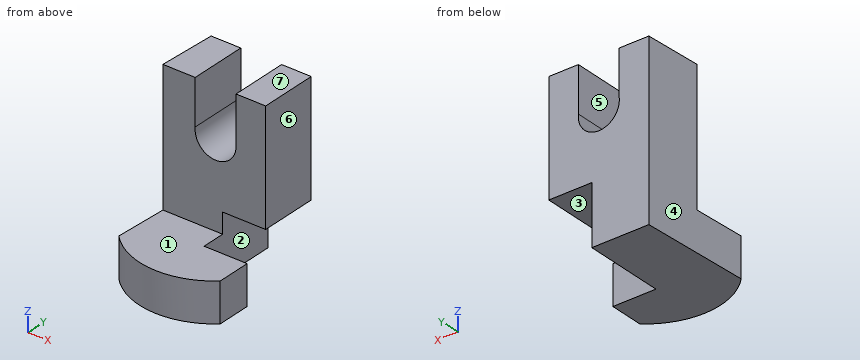
from build123d import *

# Parameters (mm, degrees)
F0_R      = 45.0325126913
F1_DEPTH  = 101.6
F3_DEPTH  = 78.486
F5_DEPTH  = 107.188
F7_DEPTH  = 186.944
F8_R      = 12.1282777673
F9_DEPTH  = 81.026
F10_W     = 24.1107804074
F10_H     = 34.6709556208
F11_DEPTH = 128.778
F13_DEPTH = 25.4
F14_W     = 27.1864784881
F14_H     = 35.0537188351
F15_DEPTH = 25.4


with BuildPart() as f1:
    # F0 (on Top) → F1 (new body)
    with BuildSketch(Plane.XY):
        Circle(F0_R)
    extrude(amount=F1_DEPTH)

    # F2 (on face) → F3 (cut)
    with BuildSketch(Plane.XY.offset(101.6)):
        Polygon((45.0325126913, 0), (-45.0325126913, 0), (-69.5492550731, 0), (45.0325126913, -116.2401661277), (161.6928875446, -116.2401661277), align=None)
    extrude(amount=-F3_DEPTH, mode=Mode.SUBTRACT)

    # F4 (on face) → F5 (cut)
    with BuildSketch(Plane.XY.offset(101.6)):
        Polygon((-61.1385696894, -57.6286986393), (-33.8673712273, -58.9006000359), (-28.4030238845, 58.2620206293), (-55.6742223466, 59.5339220259), align=None)
    extrude(amount=-F5_DEPTH, mode=Mode.SUBTRACT)

    # F6 (on face) → F7 (cut)
    with BuildSketch(Plane.XY.offset(101.6)):
        Polygon((-29.5348406238, 53.1750321388), (-29.5348406238, 33.9944170212), (29.5348406238, 33.9944170212), (29.5348406238, -32.5324498117), (45.0325126913, -32.5324498117), (45.0325126913, 59.2755898833), align=None)
    extrude(amount=-F7_DEPTH, mode=Mode.SUBTRACT)

    # F8 (on face) → F9 (cut)
    with BuildSketch(Plane.XZ):
        with Locations((0, 73.5739916563)):
            Circle(F8_R)
    extrude(amount=-F9_DEPTH, mode=Mode.SUBTRACT)

    # F10 (on face) → F11 (cut)
    with BuildSketch(Plane.XZ):
        with Locations((0, 89.5818066187)):
            Rectangle(F10_W, F10_H)
    extrude(amount=-F11_DEPTH, mode=Mode.SUBTRACT)

    # F12 (on face) → F13 (cut)
    with BuildSketch(Plane.YZ.offset(29.5348406238)):
        Polygon((0, -13.3575685322), (-16.2662249058, 23.114), (-67.4354508519, 30.6860208511), (-70.5883606289, 9.3796937905), (-70.5883606289, -6.5510598943), align=None)
    extrude(amount=F13_DEPTH, mode=Mode.SUBTRACT)

    # F14 (on face) → F15 (cut)
    with BuildSketch(Plane.YZ.offset(29.5348406238)):
        with Locations((-0.2370146103, 17.5268594176)):
            Rectangle(F14_W, F14_H)
        Polygon((13.3562246338, 35.0537188351), (13.3562246338, 0), (19.999248907, 0), (53.7981726229, 0), (53.7981726229, 35.0537188351), align=None)
    extrude(amount=-F15_DEPTH, mode=Mode.SUBTRACT)


solid = f1.part
Design review of the part built by this model. Coordinates are the model's own, in mm. Face numbers are marked on the shaded views. A direction names the side the tool comes from. Coordinates: 2 decimals unless noted, no trailing zeros. Write each loop counter-clockwise with the first axis right and the second up, starting at its lowest first coordinate (ties: lowest second). Pieces come first, ordered by that corner, then holes. Notation, with made-up numbers: (22, 27) - (53, 27) arc R25 cw to (53, 63) - close; hole circle Ø9 at (61, 45.5). An arc over 180 degrees is marked (long way). One line per item, written item: value.
1) Insertion check: pin 1 (4 mm diameter, centred on x = -11, z = 84.5, fed in from -Y); pin 2 (3 mm diameter, centred on y = 23.5, z = 81, fed in from -X); pin 3 (3 mm diameter, centred on x = -24.5, y = -19.5, fed in from +Z). Each pin has a flat end and moves straight along its axis. Give the tip position at first contact, or say it passes through.
Answer sheet:
pin 1: stops at y = 0
pin 2: stops at x = -30.09
pin 3: stops at z = 23.11
2) Add section A-A (z = 66). State the section outline as (x, y) points, plus the area to 3 significant figures.
Answer sheet:
outline: (-31.12, 0) - (-9.47, 0) - (-9.47, 33.99) - (-29.53, 33.99) - close; (9.47, 0) - (29.53, 0) - (29.53, 33.99) - (9.47, 33.99) - close
area: 1,390 mm2
3) Add section C-C (x = 0). State the section outline as (y, z) points.
Answer sheet:
outline: (-45.03, 0) - (33.99, 0) - (33.99, 61.45) - (0, 61.45) - (0, 23.11) - (-45.03, 23.11) - close
4) Mouldability with a two-part tool opening along X and no side actions: class the marked faces 4, 5, 6 and 7 as +X half, -X half, draft (parallel to the pull), parting line (faces both ways), or undercut.
Answer sheet:
face 4: -X half
face 5: undercut
face 6: +X half
face 7: draft
5) For the marked faces 1, 2 and 3, list the 3-axis set-ups (+Z, -Z, +X, -X, +Y, -Y) from which the entire face can be reached by the end or side of a thin tool; tool diameter is ignored.
Answer sheet:
face 1: +Z, +X, -X, -Y
face 2: -Z, +X, +Y
face 3: -Z, +X, +Y, -Y
6) Add section B-B (x = 10.5). State the section outline as (y, z) points, plus the area to 3 significant figures.
Answer sheet:
outline: (-43.79, 0) - (-13.83, 0) - (-13.83, 23.11) - (-43.79, 23.11) - close; (0, 35.05) - (33.99, 35.05) - (33.99, 67.5) - (0, 67.5) - close
area: 1,800 mm2
7) To check wall thickness, follow probe 1 along Z at (x, y) = (17.5, 16); probe 2 along X at (y, z) = (5.5, 83); probe 3 along Y at (x, z) = (-20.5, 68.5). State the ranges of each line that lie inside material, in increasing order.
Answer sheet:
probe 1: z = 35.05 to 101.6
probe 2: x = -30.86 to -12.06, 12.06 to 29.53
probe 3: y = 0 to 33.99
8) Add section D-D (y = 8). State the section outline as (x, z) points, plus the area to 3 significant figures.
Answer sheet:
outline: (-30.75, 0) - (4.13, 0) - (4.13, 35.05) - (29.53, 35.05) - (29.53, 101.6) - (12.06, 101.6) - (12.06, 74.9) arc R12.13 cw (long way) to (-12.06, 74.9) - (-12.06, 101.6) - (-30.75, 101.6) - close
area: 4,330 mm2
